```python
from build123d import *

# Parameters (mm, degrees)
F0_W     = 76.2
F0_H     = 38.1
F0_W_2   = 70.2
F0_H_2   = 32.1
F1_DEPTH = 42
F2_R     = 2.5
F2_R_2   = 12
F3_DEPTH = 5
F4_R     = 4.5
F5_DEPTH = 5
F7_D     = 5
F7_DEPTH = 10


with BuildPart() as f1:
    # F0 (on Front) → F1 (new body)
    with BuildSketch(Plane.XZ):
        with Locations((38.1, 19.05)):
            Rectangle(F0_W, F0_H)
        with Locations((38.1, 19.05)):
            Rectangle(F0_W_2, F0_H_2, mode=Mode.SUBTRACT)
    extrude(amount=F1_DEPTH)

    # F2 (on face) → F3 (cut)
    with BuildSketch(Plane.XY.offset(3)):
        with Locations((53.6, -5.35)):
            Circle(F2_R)
        with Locations((53.6, -36.35)):
            Circle(F2_R)
        with Locations((22.6, -36.35)):
            Circle(F2_R)
        with Locations((22.6, -5.35)):
            Circle(F2_R)
        with Locations((38.1, -20.85)):
            Circle(F2_R_2)
    extrude(amount=-F3_DEPTH, mode=Mode.SUBTRACT)

    # F4 (on face) → F5 (cut)
    with BuildSketch(Plane(origin=(0, 0, 35.1), x_dir=(1, 0, 0), z_dir=(0, 0, -1))):
        with Locations((38.1, 20.85)):
            Circle(F4_R)
    extrude(amount=-F5_DEPTH, mode=Mode.SUBTRACT)

    # F7
    with Locations(Plane.XY.offset(38.1)):
        with Locations((19.85, -20.85), (56.35, -20.85)):
            Hole(F7_D / 2, depth=F7_DEPTH)


solid = f1.part
```
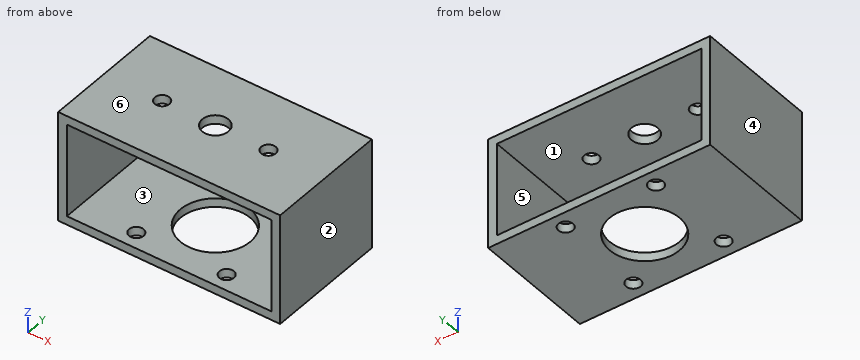
Input: part model. Units: mm. Frame: model coordinates. Face numbers are marked on the shaded views. A direction names the side the tool comes from. Coordinates: 2 decimals unless noted, no trailing zeros. Loops run counter-clockwise (first coordinate to the right, second up) from the corner with the lowest first, then second, coordinate; pieces in that order, holes last. Notation, with made-up numbers: M -37,72 L 8,72 A19 cw 8,78 Z; hole C -10,53.25 d11. An arc over 180 degrees is marked long. Answer in a Markdown table with one row per item.
1. Draft query along Z for the marked faces 3, 4, 5 and 6. Return one class per face: pulls with the +Z half, pulls with the -Z half, needs draft (parallel to the pull), parting line crosses it, or undercut.
Response:
| item | result |
|---|---|
| face 3 | undercut |
| face 4 | needs draft |
| face 5 | undercut |
| face 6 | pulls with the +Z half |
2. Material intervals for line 1 (X direction, y = -5.5, z = 2); line 2 (Z direction, x = 72, y = -4); line 3 (Y direction, x = 22, z = 1), sorted ascending.
Response:
| item | result |
|---|---|
| line 1 | x = 0 to 20.1, 25.1 to 51.1, 56.1 to 76.2 |
| line 2 | z = 0 to 3, 35.1 to 38.1 |
| line 3 | y = -42 to -38.78, -33.92 to -7.78, -2.92 to 0 |
3. Section D-D, the plane y = -20.85. Output: boundary loops of the cut face in (x, z), then the cut area to 3 significant figures.
Response:
| item | result |
|---|---|
| outline | M 0,0 L 26.1,0 L 26.1,3 L 3,3 L 3,35.1 L 17.35,35.1 L 17.35,38.1 L 0,38.1 Z; M 22.35,35.1 L 33.6,35.1 L 33.6,38.1 L 22.35,38.1 Z; M 42.6,35.1 L 53.85,35.1 L 53.85,38.1 L 42.6,38.1 Z; M 50.1,0 L 76.2,0 L 76.2,38.1 L 58.85,38.1 L 58.85,35.1 L 73.2,35.1 L 73.2,3 L 50.1,3 Z |
| area | 521 mm2 |
4. First-contact query: pin 1 (5 mm diameter, centred on x = 40, y = -26, fed in from -Z); pin 2 (4 mm diameter, centred on x = 19.85, y = -20.85, fed in from +Z). Flat tips, straight axial feed; report the tip coordinate or a pass-through.
Response:
| item | result |
|---|---|
| pin 1 | stops at z = 35.1 |
| pin 2 | stops at z = 3 |
5. Section A-A, the plane y = -36.35. Output: boundary loops of the cut face in (x, z), then the cut area to 3 significant figures.
Response:
| item | result |
|---|---|
| outline | M 0,0 L 20.1,0 L 20.1,3 L 3,3 L 3,35.1 L 73.2,35.1 L 73.2,3 L 56.1,3 L 56.1,0 L 76.2,0 L 76.2,38.1 L 0,38.1 Z; M 25.1,0 L 51.1,0 L 51.1,3 L 25.1,3 Z |
| area | 620 mm2 |
6. Reachability of the marked faces 1 and 2 from +Z, -Z, +X, -X, +Y, -Y: full face, straight path, thin tool, end or side. Return the list, or none.
Response:
| item | result |
|---|---|
| face 1 | +Y, -Y |
| face 2 | +Z, -Z, +X, +Y, -Y |
7. Section C-C, the plane x = 37. Output: boundary loops of the cut face in (y, z).
Response:
| item | result |
|---|---|
| outline | M -42,0 L -32.8,0 L -32.8,3 L -42,3 Z; M -42,35.1 L -25.21,35.1 L -25.21,38.1 L -42,38.1 Z; M -16.49,35.1 L 0,35.1 L 0,38.1 L -16.49,38.1 Z; M -8.9,0 L 0,0 L 0,3 L -8.9,3 Z |
8. Section B-B, the plane z = 4.5. Output: boundary loops of the cut face in (x, y).
Response:
| item | result |
|---|---|
| outline | M 0,-42 L 3,-42 L 3,0 L 0,0 Z; M 73.2,-42 L 76.2,-42 L 76.2,0 L 73.2,0 Z |
